```python
from build123d import *

# Parameters (mm, degrees)
SKETCH1_W           = 34
SKETCH1_H           = 12
BOSS_EXTRUDE1_DEPTH = 5
SKETCH5_R           = 3
BOSS_EXTRUDE3_DEPTH = 7
SKETCH6_R           = 1.5
CUT_EXTRUDE1_DEPTH  = 3
SKETCH8_R           = 4
CUT_EXTRUDE4_DEPTH  = 87.890735985


with BuildPart() as part:
    # Sketch1 → Boss-Extrude1 (new body)
    with BuildSketch(Plane(origin=(0, 0, 0), x_dir=(1, 0, 0), z_dir=(0, 1, 0))):
        Rectangle(SKETCH1_W, SKETCH1_H)
    extrude(amount=BOSS_EXTRUDE1_DEPTH)

    # Sketch5 → Boss-Extrude3 (add)
    with BuildSketch(Plane(origin=(17, 0, 0), x_dir=(0, 0, -1), z_dir=(1, 0, 0))):
        with BuildLine():
            Line((-6, 5), (6, 5))
            Line((6, 5), (6, 84))
            ThreePointArc((6, 84), (0, 90), (-6, 84))
            Line((-6, 84), (-6, 5))
        make_face()
        with Locations((0, 84)):
            Circle(SKETCH5_R, mode=Mode.SUBTRACT)
        with Locations((-0.5, 63.5)):
            Circle(SKETCH5_R, mode=Mode.SUBTRACT)
    boss_extrude3 = extrude(amount=-BOSS_EXTRUDE3_DEPTH)

    # Sketch6 → Cut-Extrude1 (cut)
    with BuildSketch(Plane(origin=(0, 5, 0), x_dir=(1, 0, 0), z_dir=(0, 1, 0))):
        with Locations(Location((0, 0, 0), (0, 0, 270))):
            Circle(SKETCH6_R)
    extrude(amount=-CUT_EXTRUDE1_DEPTH, mode=Mode.SUBTRACT)

    # Sketch8 → Cut-Extrude4 (cut, through all)
    with BuildSketch(Plane(origin=(0, 5, 0), x_dir=(1, 0, 0), z_dir=(0, 1, 0))):
        with Locations(Location((0, 0, 0), (0, 0, 270))):
            Circle(SKETCH8_R)
    extrude(amount=-CUT_EXTRUDE4_DEPTH, mode=Mode.SUBTRACT)

    # Mirror1: Boss-Extrude3 across plane
    add(boss_extrude3.mirror(Plane(origin=(0, 0, 0), x_dir=(0, 0, 1), z_dir=(1, 0, 0))))


solid = part.part
```
Source: CAD feature listing. Evaluate the final solid. Frame: model axes, mm. A direction names the side the tool comes from. Give positions to 0.01 mm unless a question says otherwise; leave off trailing zeros. Order: outer loops, then holes, each group sorted by start corner. A loop starts at its lowest first (then second) coordinate and runs counter-clockwise, first axis right, second up. Notation, with made-up numbers: (-20, 73.5) -> (28, 73.5) arc R19 ccw to (28, 89.5) -> close; hole circle Ø1 at (69, -6). An arc over 180 degrees is marked (long way). Use a Markdown table: item, result.
Q1. Access query for faces 4 (the face through (-13.55, 81.07, 0.65)), 5 (the face through (10, 48, 0)). Directions: +Z, -Z, +X, -X, +Y, -Y. A direction counts if a zero-diameter tool reaches every point of the face in a straight line with its end or side. Return the directions, or none.
A:
| item | result |
|---|---|
| face 4 | +X, -X |
| face 5 | +Z, -Z, +Y |
Q2. First-contact query: P1, Ø6, axis at x = 3, z = 1.5, coming from the +Y side; P2, Ø3.5, axis at y = 63.5, z = 0.5, coming from the +X side (3 decimals). Flat tips, straight axial feed; report the tip coordinate or a pass-through.
A:
| item | result |
|---|---|
| P1 | y = 5 |
| P2 | through |
Q3. Section B-B (x = 0). Return the cut outline in (y, z), and give its area (3 significant figures).
A:
| item | result |
|---|---|
| outline | (0, -6) -> (5, -6) -> (5, -4) -> (0, -4) -> close; (0, 4) -> (5, 4) -> (5, 6) -> (0, 6) -> close |
| area | 20.0 mm^2 |
Q4. Section D-D (x = 11.5). Return the cut outline in (y, z).
A:
| item | result |
|---|---|
| outline | (0, -6) -> (84, -6) arc R6 ccw to (84, 6) -> (0, 6) -> close; hole circle Ø6 at (63.5, 0.5); hole circle Ø6 at (84, 0) |
Q5. Section A-A (y = 55). Return the cut outline in (x, z), and give its area (3 significant figures).
A:
| item | result |
|---|---|
| outline | (-17, -6) -> (-10, -6) -> (-10, 6) -> (-17, 6) -> close; (10, -6) -> (17, -6) -> (17, 6) -> (10, 6) -> close |
| area | 168 mm^2 |
Q6. Material intervals for line 1 (X direction, y = 71.5, z = 2.5); line 2 (Y direction, x = -12, z = 0); line 3 (Y direction, x = -9, z = -5.5), sorted ascending. Write a range as [from, to].
A:
| item | result |
|---|---|
| line 1 | [-17, -10], [10, 17] |
| line 2 | [0, 60.54], [66.46, 81], [87, 90] |
| line 3 | [0, 5] |
Q7. Pull-direction query (Z, two-part tool) for faces 1 (the face through (4.3, 5, -0.1)), 2 (the face through (14, 90, 0)), 3 (the face through (-3.905, 2.535, -0.867)); classes: +Z half, -Z half, draft (parallel to the pull), parting line (faces both ways), or undercut.
A:
| item | result |
|---|---|
| face 1 | draft |
| face 2 | parting line |
| face 3 | undercut |
Q8. Section C-C (z = 1.5). Return the cut outline in (x, y), and give its area (3 significant figures).
A:
| item | result |
|---|---|
| outline | (-17, 0) -> (-3.71, 0) -> (-3.71, 5) -> (-10, 5) -> (-10, 60.67) -> (-17, 60.67) -> close; (-17, 66.33) -> (-10, 66.33) -> (-10, 81.4) -> (-17, 81.4) -> close; (-17, 86.6) -> (-10, 86.6) -> (-10, 89.81) -> (-17, 89.81) -> close; (3.71, 0) -> (17, 0) -> (17, 60.67) -> (10, 60.67) -> (10, 5) -> (3.71, 5) -> close; (10, 66.33) -> (17, 66.33) -> (17, 81.4) -> (10, 81.4) -> close; (10, 86.6) -> (17, 86.6) -> (17, 89.81) -> (10, 89.81) -> close |
| area | 1,170 mm^2 |
